```python
from build123d import *

# Parameters (mm, degrees)
F0_R           = 123.825
F1_DEPTH       = 25.4
F3_R           = 123.825
F4_DEPTH       = 25.4
F5_R           = 123.825
F5_R_2         = 111.125
F6_DEPTH       = 609.6
F7_R           = 136.525
F8_DEPTH       = 25.4
F9_W           = 25.4
F9_H           = 274.828
F11_W          = 82.042
F11_H          = 10.16
F12_DEPTH      = 228.601
F12_DEPTH_BACK = 228.601


with BuildPart() as f1:
    # F0 (on Top) → F1 (new body)
    with BuildSketch(Plane.XY):
        with BuildLine():
            ThreePointArc((151.5545215542, -154.6173465054), (229.3385530798, -94.074537579), (258.7625, 0))
            ThreePointArc((258.7625, 0), (229.3385530798, 94.074537579), (151.5545215542, 154.6173465054))
            Line((151.5545215542, 154.6173465054), (-46.0375, 228.6))
            Line((-46.0375, 228.6), (-122.2375, 228.6))
            Line((-122.2375, 228.6), (-122.2375, 0))
            Line((-122.2375, 0), (-122.2375, -228.6))
            Line((-122.2375, -228.6), (-46.0375, -228.6))
            Line((-46.0375, -228.6), (151.5545215542, -154.6173465054))
        make_face()
        with Locations((93.6625, 0)):
            Circle(F0_R, mode=Mode.SUBTRACT)
    extrude(amount=-F1_DEPTH)



with BuildPart() as f4:
    # F3 (on offset) → F4 (new body)
    with BuildSketch(Plane.XY.offset(-325.628)):
        with BuildLine():
            Line((-46.0375, -228.6), (151.5545215542, -154.6173465054))
            ThreePointArc((151.5545215542, -154.6173465054), (258.7625, 0), (151.5545215542, 154.6173465054))
            Line((151.5545215542, 154.6173465054), (-46.0375, 228.6))
            Line((-46.0375, 228.6), (-122.2375, 228.6))
            Line((-122.2375, 228.6), (-122.2375, -228.6))
            Line((-122.2375, -228.6), (-46.0375, -228.6))
        make_face()
        with Locations((93.6625, 0)):
            Circle(F3_R, mode=Mode.SUBTRACT)
    extrude(amount=F4_DEPTH)


with BuildPart() as f1_1:
    add(f1.part)

    add(f4.part)  # F6 merges F4
    # F5 (on face) → F6 (join)
    with BuildSketch(Plane.XY):
        with Locations((93.6625, 0)):
            Circle(F5_R)
        with Locations((93.6625, 0)):
            Circle(F5_R_2, mode=Mode.SUBTRACT)
    extrude(amount=-F6_DEPTH)

    # F7 (on face) → F8 (join)
    with BuildSketch(Plane(origin=(0, 0, -609.6), x_dir=(1, 0, 0), z_dir=(0, 0, -1))):
        with Locations((93.6625, 0)):
            Circle(F7_R)
    extrude(amount=F8_DEPTH)

    # F9 (on face) → F10 (join, up to the next surface of F1)
    with BuildSketch(Plane(origin=(-122.2375, 0, 0), x_dir=(0, -1, 0), z_dir=(-1, 0, 0))):
        with Locations((0, -162.814)):
            Rectangle(F9_W, F9_H)
    extrude(until=Until.NEXT, dir=(1, 0, 0))

    # F11 (on Front) → F12 (cut, two sides)
    with BuildSketch(Plane.XZ) as f12_sk:
        with Locations((-81.2165, -30.48)):
            Rectangle(F11_W, F11_H)
    extrude(amount=-F12_DEPTH, mode=Mode.SUBTRACT)
    extrude(f12_sk.sketch, amount=F12_DEPTH_BACK, mode=Mode.SUBTRACT)


solid = f1_1.part
```
Design review of the part built by this model. Coordinates are the model's own, in mm. A direction names the side the tool comes from. Round coordinates to 2 decimals unless told otherwise and drop trailing zeros. Write each loop counter-clockwise with the first axis right and the second up, starting at its lowest first coordinate (ties: lowest second). Pieces come first, ordered by that corner, then holes. Notation, with made-up numbers: (18.5, -22.5) -> (69.5, -22.5) arc R27 ccw to (69.5, 11.5) -> close; hole circle Ø4 at (-23.75, 47.25). An arc over 180 degrees is marked (long way). Answer in a Markdown table with one row per item.
Q1. Draft analysis for pull direction Z (two halves, no side actions). For faces 1 (the face through (123, 121, -609.6)), 2 (the face through (-122.238, 1, -267)), 3 (the face through (-19, 3, 0)), 4 (the face through (-82, 0, -35.56)), state which applies: +Z half, -Z half, draft (parallel to the pull), parting line (faces both ways), or undercut.
The answers:
| item | result |
|---|---|
| face 1 | undercut |
| face 2 | draft |
| face 3 | +Z half |
| face 4 | undercut |
Q2. Take a section at D-D, the plane x = 66. State the section outline as (y, z) points, then the cut area to 3 significant figures.
The answers:
| item | result |
|---|---|
| outline | (-186.65, -325.63) -> (-120.7, -325.63) -> (-120.7, -609.6) -> (-133.69, -609.6) -> (-133.69, -635) -> (133.69, -635) -> (133.69, -609.6) -> (120.7, -609.6) -> (120.7, -325.63) -> (186.65, -325.63) -> (186.65, -300.23) -> (120.7, -300.23) -> (120.7, -25.4) -> (186.65, -25.4) -> (186.65, 0) -> (107.63, 0) -> (107.63, -609.6) -> (-107.63, -609.6) -> (-107.63, 0) -> (-186.65, 0) -> (-186.65, -25.4) -> (-120.7, -25.4) -> (-120.7, -300.23) -> (-186.65, -300.23) -> close |
| area | 29,400 mm² |
Q3. Take a section at C-C, the plane y = 200.5. State the section outline as (x, z) points.
The answers:
| item | result |
|---|---|
| outline | (-122.24, -325.63) -> (29.01, -325.63) -> (29.01, -300.23) -> (-122.24, -300.23) -> close; (-122.24, -25.4) -> (29.01, -25.4) -> (29.01, 0) -> (-122.24, 0) -> close |
Q4. For faces 5 (the face through (-4.601, -75.346, -465.626)), 6 (the face through (79.2, 110.18, -300.53)), 7 (the face through (-14.68, 83.07, -622.12)), list the 3-axis set-ups (+Z, -Z, +X, -X, +Y, -Y) from which the entire face can be reached by the end or side of a thin tool; tool diameter is ignored.
The answers:
| item | result |
|---|---|
| face 5 | none |
| face 6 | +Z |
| face 7 | -Z |
Q5. Clearance check with flat-ended pins moving along their axes: pin 1 Ø2 at (x, y) = (34.5, 135) entering from -Z; pin 2 Ø5 at (y, z) = (-6, -29.5) entering from -X; pin 3 Ø2 at (y, z) = (41, -546.5) entering from +X; pin 4 Ø5 at (y, z) = (-127, -461) entering from +X. State where each tip first meets the part, or that it passes through.
The answers:
| item | result |
|---|---|
| pin 1 | z = -325.63 |
| pin 2 | x = -40.2 |
| pin 3 | x = 210.85 |
| pin 4 | through |
Q6. Take a section at A-A, the plane x = -83. State the section outline as (y, z) points, then the cut area to 3 significant figures.
The answers:
| item | result |
|---|---|
| outline | (-228.6, -325.63) -> (228.6, -325.63) -> (228.6, -300.23) -> (12.7, -300.23) -> (12.7, -35.56) -> (-12.7, -35.56) -> (-12.7, -300.23) -> (-228.6, -300.23) -> close; (-228.6, -25.4) -> (228.6, -25.4) -> (228.6, 0) -> (-228.6, 0) -> close |
| area | 29,900 mm² |
Q7. To check wall thickness, follow L1, parallel to Z at x = 224.5, y = -14; L2, parallel to Z at x = 165.5, y = -117; L3, parallel to X at y = 6, z = -396.5. State the ranges of each line that lie inside material, in increasing order. Write a range as [from, to].
The answers:
| item | result |
|---|---|
| L1 | [-635, -609.6], [-325.63, -300.23], [-25.4, 0] |
| L2 | [-325.63, -300.23], [-25.4, 0] |
| L3 | [-30.02, -17.3], [204.63, 217.34] |
